from build123d import *

# Parameters (mm, degrees)
SKETCH1_W           = 41.256811376
SKETCH1_H           = 15.875111739
SKETCH1_R           = 3
BOSS_EXTRUDE1_DEPTH = 5
SKETCH2_W           = 41.256811376
SKETCH2_H           = 15
BOSS_EXTRUDE3_DEPTH = 5
SKETCH3_W           = 41.256811376
SKETCH3_H           = 38.931242613
SKETCH3_R           = 3
BOSS_EXTRUDE5_DEPTH = 5


with BuildPart() as part:
    # Sketch1 → Boss-Extrude1 (new body)
    with BuildSketch(Plane.XY):
        with Locations((85.088811215, -27.526454456)):
            Rectangle(SKETCH1_W, SKETCH1_H)
        with Locations((94.366601686, -27.526454455)):
            Circle(SKETCH1_R, mode=Mode.SUBTRACT)
        with Locations((75.811020744, -27.526454455)):
            Circle(SKETCH1_R, mode=Mode.SUBTRACT)
    extrude(amount=BOSS_EXTRUDE1_DEPTH)

    # Sketch2 → Boss-Extrude3 (add)
    with BuildSketch(Plane.XY.offset(5)):
        with Locations((85.088811215, -42.964010325)):
            Rectangle(SKETCH2_W, SKETCH2_H)
    extrude(amount=-BOSS_EXTRUDE3_DEPTH)

    # Sketch3 → Boss-Extrude5 (add)
    with BuildSketch(Plane.XZ.offset(50.464010325)):
        with Locations((85.088811215, 24.465621307)):
            Rectangle(SKETCH3_W, SKETCH3_H)
        with Locations(Location((76.213848726, 32.840318874, 0), (0, 0, 270))):
            Circle(SKETCH3_R, mode=Mode.SUBTRACT)
        with Locations(Location((90.760010617, 19.114096734, 0), (0, 0, 270))):
            Circle(SKETCH3_R, mode=Mode.SUBTRACT)
    extrude(amount=-BOSS_EXTRUDE5_DEPTH)


with BuildPart() as body_2:
    # Mirror1: mirrored copy
    add(part.part.mirror(Plane(origin=(64.460405527, -19.588898586, 5), x_dir=(0, 0, 1), z_dir=(0, -1, 0))))


solid = body_2.part
Can you work these out from the model? Positions are in its coordinate system, mm. A direction names the side the tool comes from. Give positions to 0.01 mm unless a question says otherwise; leave off trailing zeros. Order: outer loops, then holes, each group sorted by start corner. A loop starts at its lowest first (then second) coordinate and runs counter-clockwise, first axis right, second up. Notation, with made-up numbers: M 88.25,18.5 L 147.25,18.5 A20 ccw 147.25,35.5 Z; hole C -29.75,40.25 d9. An arc over 180 degrees is marked long. Use one line per item in the form item = value. Start each with the question number.
Item 1: If we section it at C-C (z = 34.5): Write out the boundary of the cut face in (x, y).
Item 2: For faces 4 (the flat face through (85, -7, 5)), 5 (the flat face through (105.717, 8, 14)), which set-ups out of +Z, -Z, +X, -X, +Y, -Y let a thin tool reach every point of the face, with its end or its side?
Item 3: We'd pull the mould along Z, two halves only. Please class faces 1 (the flat face through (85, -19.589, 2)), 2 (the flat face through (85, 9, 43.931)), 3 (the cylindrical face through (87.83, 8.82, 19.76)): +Z half, -Z half, draft (parallel to the pull), parting line (faces both ways), or undercut.
Item 4: If we section it at D-D (x = 86.5): Write out the boundary of the cut face in (y, z).
Item 5: If I drill on line 1 along X through (y, z) = (-14, 4); line 2 along Y through (x, z) = (70.5, 9.5); line 3 along Z through (x, y) = (78, -8.5), over which ranges is the centre line in solid material (lowest first)?
Item 6: If we section it at B-B (x = 74): Write out the boundary of the cut face in (y, z), then the cut area to 3 significant figures.
Item 7: If we section it at A-A (y = -10): Write out the boundary of the cut face in (x, z).
Item 8: Will these pins go through, and if not, where does the flat tip stop? pin 1 Ø12 at (x, y) = (88, -12.5) entering from -Z; pin 2 Ø11.5 at (x, z) = (89.5, 16.5) entering from -Y; pin 3 Ø5 at (x, y) = (75.81, -11.65) entering from +Z; pin 4 Ø1 at (x, y) = (88.5, 5) entering from +Z.
Outcome:
q1.outline = M 64.46,6.29 L 73.71,6.29 L 73.71,11.29 L 64.46,11.29 Z; M 78.71,6.29 L 105.72,6.29 L 105.72,11.29 L 78.71,11.29 Z
q2.face_4 = +Z, +X, -X, -Y
q2.face_5 = +Z, -Z, +X, +Y, -Y
q3.face_1 = draft
q3.face_2 = +Z half
q3.face_3 = undercut
q4.outline = M -19.59,0 L 11.29,0 L 11.29,43.93 L 6.29,43.93 L 6.29,5 L -19.59,5 Z
q5.line_1 = 64.46 to 73.94, 77.68 to 92.5, 96.23 to 105.72
q5.line_2 = 6.29 to 11.29
q5.line_3 = 0 to 5
q6.outline = M -19.59,0 L -14.04,0 L -14.04,5 L -19.59,5 Z; M -9.26,0 L 11.29,0 L 11.29,30.82 L 6.29,30.82 L 6.29,5 L -9.26,5 Z; M 6.29,34.86 L 11.29,34.86 L 11.29,43.93 L 6.29,43.93 Z
q6.area = 305 mm2
q7.outline = M 64.46,0 L 73.31,0 L 73.31,5 L 64.46,5 Z; M 78.32,0 L 91.86,0 L 91.86,5 L 78.32,5 Z; M 96.87,0 L 105.72,0 L 105.72,5 L 96.87,5 Z
q8.pin_1 = 0
q8.pin_2 = 6.29
q8.pin_3 = through
q8.pin_4 = 5
